Autodesk Inventor part; units mm, degrees
ref_plane "Work Plane1" through (0, 0, 7.62) normal (0, 0, 1) x (1, 0, 0)
ref_plane "YZ Plane" through (0, 0, 0) normal (1, 0, 0) x (0, 1, 0)
ref_plane "XZ Plane" through (0, 0, 0) normal (0, 1, 0) x (-1, 0, 0)
sketch "Sketch1" plane through (0, 0, 0) normal (0, 1, 0) x (-1, 0, 0)
  circle A0 centre (0, 7.62) radius 0.535
  point P0 (0, 0)
  dimension "d0" = 1.07
  dimension "d1" = 7.62
extrude "Extrusion1" add sketch "Sketch1" along normal blind 3.94
ref_plane "Work Plane1" through (0, 0, 7.62) normal (0, 0, 1) x (1, 0, 0)
sketch "Sketch2" plane through (0, 0, 7.62) normal (0, 0, 1) x (1, 0, 0)
  line L0 (-0.95, 4.94) -> (0.95, 4.94)
  line L1 (0.95, 4.94) -> (0.95, 3.94)
  line L2 (0.95, 3.94) -> (-0.95, 3.94)
  line L3 (-0.95, 3.94) -> (-0.95, 4.94)
  line L4 (-0.535, 0) -> (0.535, 0)
  line L5 (0, 0) -> (0, -0.058)
  dimension "d5" = 3.94
  dimension "d6" = 1.9
  dimension "d7" = 0.95
  dimension "d8" = 1
extrude "Extrusion2" add sketch "Sketch2" along normal mid plane 0.6
fillet "Fillet1" radius 0.2 4 edges at (0.95, 3.94, 7.62) (0.95, 4.94, 7.62) (-0.95, 4.94, 7.62) (-0.95, 3.94, 7.62)
sketch "Sketch3" plane through (-0.75, 4.94, 7.92) normal (0, 1, 0) x (1, 0, 0)
  circle A0 centre (0.75, 0.3) radius 0.535
  point P0 (0.75, 7.92)
  dimension "d12" = 1.07
  dimension "d13" = 7.62
extrude "Extrusion3" add sketch "Sketch3" along normal blind 0.6
sketch "Sketch4" plane through (0, 5.54, 7.62) normal (0, 1, 0) x (1, 0, 0)
  line L0 (0.75, 0.3) -> (0.95, 0.3)
  line L1 (-0.95, -0.3) -> (0.95, -0.3)
  line L2 (0.95, -0.3) -> (0.95, 0.3)
  line L3 (0.95, 0.3) -> (-0.95, 0.3)
  line L4 (-0.95, 0.3) -> (-0.95, -0.3)
  point P0 (0, 7.62)
sketch "Sketch5" plane through (0, 0, 0) normal (1, 0, 0) x (0, 1, 0)
  line L0 (27.34, 0) -> (27.34, 5.62)
  line L1 (3.94, 7.085) -> (3.94, 7.32)
  line L2 (5.54, 7.085) -> (5.54, 8.155)
  line L3 (5.54, 7.62) -> (25.34, 7.62)
  arc A0 (27.34, 5.62) -> (25.34, 7.62) centre (25.34, 5.62) ccw
  point P0 (0, 0)
  dimension "d16" = 23.4
  dimension "d17" = 2
sweep "Sweep1" add profiles "Sketch4" path "Sketch5" path curves L3 A0 L0
mirror "Mirror1" about plane through (0, 0, 0) normal (0, 0, 1) of "Sweep1", "Extrusion3", "Fillet1", "Extrusion2", "Extrusion1"
ref_plane "Work Plane2" through (0, 0, -7.62) normal (0, 0, 1) x (1, 0, 0)
properties part number "OAR3R010FLF_CurrentSense"
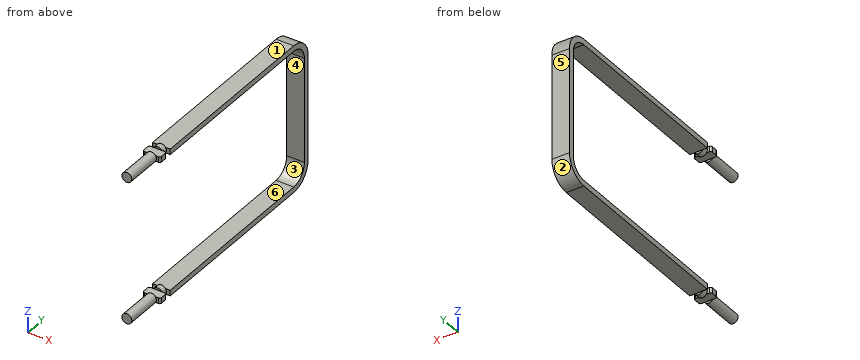
The listing builds one solid part. Answer for the finished solid, in the listing's coordinates (mm). Face numbers are marked on the shaded views. A direction names the side the tool comes from. Coordinates: 2 decimals unless noted, no trailing zeros. Order: outer loops, then holes, each group sorted by start corner. A loop starts at its lowest first (then second) coordinate and runs counter-clockwise, first axis right, second up.
Q1. A cutting plane is placed at B-B, the plane z = -3. Write down the section's boundary in (x, y), and give its area (3 significant figures).
Q2. A cutting plane is placed at A-A, the plane y = 18.25. Write down the section's boundary in (x, z), and give its area (3 significant figures).
Q3. Given P1, Ø0.5, axis at x = -0.5, y = 4, coming from the -Z side; P2, Ø0.6, axis at x = 0, y = 19.5, coming from the -Z side; P3, Ø1, axis at x = 0, y = 11.5, coming from the +Z side, each flat-ended and moving along its own axis, determine where each tip first touches the part or whether it passes through.
Q4. A cutting plane is placed at C-C, the plane z = 7.62. Write down the section's boundary in (x, y) (3 decimals), and give its area (3 significant figures).
Q5. For a pull along Y with two mould halves and no side action, classify the marked faces 4, 5 and 6 as pulls with the +Y half, pulls with the -Y half, needs draft (parallel to the pull), parting line crosses it, or undercut.
Q6. Consider line 1 (Z direction, x = 0.15, y = 23); line 2 (Z direction, x = 0.05, y = 5.25); line 3 (Y direction, x = 0.45, z = 4.5). Determine where each line is inside the solid, lowest interval first.
Q7. Which of the six approach directions +Z, -Z, +X, -X, +Y, -Y give full straight-line access (tool end or side, diameter ignored) to the marked faces 1, 2 and 3?
Answers follow:
1. outline: (-0.95, 27.04) - (0.95, 27.04) - (0.95, 27.64) - (-0.95, 27.64) - close
1. area: 1.14 mm2
2. outline: (-0.95, -7.92) - (0.95, -7.92) - (0.95, -7.32) - (-0.95, -7.32) - close; (-0.95, 7.32) - (0.95, 7.32) - (0.95, 7.92) - (-0.95, 7.92) - close
2. area: 2.28 mm2
3. P1: stops at z = -8.09
3. P2: stops at z = -7.92
3. P3: stops at z = 7.92
4. outline: (-0.95, 4.14) arc R0.2 ccw to (-0.75, 3.94) - (-0.535, 3.94) - (-0.535, 0) - (0.535, 0) - (0.535, 3.94) - (0.75, 3.94) arc R0.2 ccw to (0.95, 4.14) - (0.95, 4.74) arc R0.2 ccw to (0.75, 4.94) - (0.535, 4.94) - (0.535, 5.54) - (0.95, 5.54) - (0.95, 26.476) - (-0.95, 26.476) - (-0.95, 5.54) - (-0.535, 5.54) - (-0.535, 4.94) - (-0.75, 4.94) arc R0.2 ccw to (-0.95, 4.74) - close
4. area: 46.5 mm2
5. face 4: pulls with the -Y half
5. face 5: pulls with the +Y half
5. face 6: undercut
6. line 1: z = -7.92 to -7.32, 7.32 to 7.92
6. line 2: z = -8.15 to -7.09, 7.09 to 8.15
6. line 3: y = 27.04 to 27.64
7. face 1: +Z, +X, -X, +Y
7. face 2: -Z, +X, -X, +Y
7. face 3: +X, -X
